```python
from build123d import *

# Parameters (mm, degrees)
MODEL_R                         = 1
MODEL_W                         = 12.3
MODEL_H                         = 22.500175579
BRIDA_BASE1_DEPTH               = 1
PLIEGUE_START                   = -94.948568727
PLIEGUE_CROQUIZADO1_DEPTH       = 36.500175579
PLIEGUE_CROQUIZADO1_2_DEPTH     = 2
PLIEGUE_START_2                 = -60.448393148
PLIEGUE_CROQUIZADO1_3_DEPTH     = 2
PLIEGUE_CROQUIZADO1_4_DEPTH     = 36.500175579
PLIEGUE_START_3                 = -92.948568727
PLIEGUE_CROQUIZADO1_5_DEPTH     = 32.500175579
PLIEGUE_START_4                 = 176.99991226
PLIEGUE_CROQUIZADO1_6_OUTLINE_R = 1
PLIEGUE_CROQUIZADO1_6_DEPTH     = 1


with BuildPart() as part:
    # Brida base1: sheet metal written as solids
    # Model → Brida base1 (new body)
    with BuildSketch(Plane.XY):
        with BuildLine():
            Line((178.265288891, -94.948568727), (178.265288891, -92.948568727))
            Line((178.265288891, -92.948568727), (177.265288891, -92.948568727))
            Line((177.265288891, -92.948568727), (177.265288891, -94.948568727))
            Line((177.265288891, -94.948568727), (169.565288891, -94.948568727))
            ThreePointArc((169.565288891, -94.948568727), (168.151075328, -94.362782289), (167.565288891, -92.948568727))
            Line((167.565288891, -92.948568727), (167.565288891, -60.448393148))
            ThreePointArc((167.565288891, -60.448393148), (168.151075328, -59.034179585), (169.565288891, -58.448393148))
            Line((169.565288891, -58.448393148), (177.265288891, -58.448393148))
            Line((177.265288891, -58.448393148), (177.265288891, -60.448393148))
            Line((177.265288891, -60.448393148), (178.265288891, -60.448393148))
            Line((178.265288891, -60.448393148), (178.265288891, -58.448393148))
            Line((178.265288891, -58.448393148), (195.565288891, -58.448393148))
            ThreePointArc((195.565288891, -58.448393148), (196.979502453, -59.034179585), (197.565288891, -60.448393148))
            Line((197.565288891, -60.448393148), (197.565288891, -92.948568727))
            ThreePointArc((197.565288891, -92.948568727), (196.979502453, -94.362782289), (195.565288891, -94.948568727))
            Line((195.565288891, -94.948568727), (178.265288891, -94.948568727))
        make_face()
        with Locations((171.565288891, -90.348568727)):
            Circle(MODEL_R, mode=Mode.SUBTRACT)
        with Locations((171.565288891, -63.048393148)):
            Circle(MODEL_R, mode=Mode.SUBTRACT)
        with Locations((188.165288891, -63.048393148)):
            Circle(MODEL_R, mode=Mode.SUBTRACT)
        with Locations((188.165288891, -90.348568727)):
            Circle(MODEL_R, mode=Mode.SUBTRACT)
        with Locations((188.415288891, -76.698480938)):
            Rectangle(MODEL_W, MODEL_H, mode=Mode.SUBTRACT)
    extrude(amount=-BRIDA_BASE1_DEPTH)

    # Pliegue croquizado1: read off the stored shape, not the designer's step
    # Pliegue croquizado1 outline → Pliegue croquizado1 (cut)
    with BuildSketch(Plane(origin=(0, 0, 0), x_dir=(1, 0, 0), z_dir=(0, 1, 0)).offset(PLIEGUE_START)):
        with BuildLine():
            Line((167.565288891, 0), (177.163871169, 0))
            ThreePointArc((177.163871169, 0), (177.804686096, 0.728828115), (178.73651226, 1))
            Line((178.73651226, 1), (167.565288891, 1))
            Line((167.565288891, 1), (167.565288891, 0))
        make_face()
    extrude(amount=PLIEGUE_CROQUIZADO1_DEPTH, mode=Mode.SUBTRACT)

    # Pliegue croquizado1 2 outline → Pliegue croquizado1 2 (cut)
    with BuildSketch(Plane(origin=(0, 0, 0), x_dir=(1, 0, 0), z_dir=(0, 1, 0)).offset(PLIEGUE_START)):
        with BuildLine():
            ThreePointArc((177.265288891, 0.186049099), (177.211739726, 0.094572835), (177.163871169, 0))
            Line((177.163871169, 0), (177.265288891, 0))
            Line((177.265288891, 0), (177.265288891, 0.186049099))
        make_face()
        Polygon((178.265288891, 0), (178.441395947, 0), (178.265288891, 0.439557056), align=None)
    extrude(amount=PLIEGUE_CROQUIZADO1_2_DEPTH, mode=Mode.SUBTRACT)

    # Pliegue croquizado1 3 outline → Pliegue croquizado1 3 (cut)
    with BuildSketch(Plane(origin=(0, 0, 0), x_dir=(1, 0, 0), z_dir=(0, 1, 0)).offset(PLIEGUE_START_2)):
        with BuildLine():
            ThreePointArc((177.265288891, 0.186049099), (177.211739726, 0.094572835), (177.163871169, 0))
            Line((177.163871169, 0), (177.265288891, 0))
            Line((177.265288891, 0), (177.265288891, 0.186049099))
        make_face()
        Polygon((178.265288891, 0), (178.441395947, 0), (178.265288891, 0.439557056), align=None)
    extrude(amount=PLIEGUE_CROQUIZADO1_3_DEPTH, mode=Mode.SUBTRACT)

    # Pliegue croquizado1 4 outline → Pliegue croquizado1 4 (add)
    with BuildSketch(Plane(origin=(0, 0, 0), x_dir=(1, 0, 0), z_dir=(0, 1, 0)).offset(PLIEGUE_START)):
        with BuildLine():
            Line((176.99991226, -9.965376631), (177.99991226, -9.965376631))
            Line((177.99991226, -9.965376631), (177.99991226, -0.7366))
            ThreePointArc((177.99991226, -0.7366), (178.01324203, -0.597101848), (178.0527489, -0.46265251))
            Line((178.0527489, -0.46265251), (177.124479337, -0.090744432))
            ThreePointArc((177.124479337, -0.090744432), (177.031338378, -0.407720702), (176.99991226, -0.7366))
            Line((176.99991226, -0.7366), (176.99991226, -9.965376631))
        make_face()
        with BuildLine():
            Line((178.441395947, 0), (178.462564769, -0.05283664))
            ThreePointArc((178.462564769, -0.05283664), (178.597014107, -0.01332977), (178.73651226, 0))
            Line((178.73651226, 0), (178.441395947, 0))
        make_face()
        with BuildLine():
            Line((178.090656691, 0.875432923), (178.265288891, 0.439557056))
            Line((178.265288891, 0.439557056), (178.265288891, 0.934844913))
            ThreePointArc((178.265288891, 0.934844913), (178.17718339, 0.907459237), (178.090656691, 0.875432923))
        make_face()
    extrude(amount=PLIEGUE_CROQUIZADO1_4_DEPTH)

    # Pliegue croquizado1 5 outline → Pliegue croquizado1 5 (add)
    with BuildSketch(Plane(origin=(0, 0, 0), x_dir=(1, 0, 0), z_dir=(0, 1, 0)).offset(PLIEGUE_START_3)):
        with BuildLine():
            Line((177.124479337, -0.090744432), (178.0527489, -0.46265251))
            ThreePointArc((178.0527489, -0.46265251), (178.215657405, -0.215745145), (178.462564769, -0.05283664))
            Line((178.462564769, -0.05283664), (178.441395947, 0))
            Line((178.441395947, 0), (177.163871169, 0))
            ThreePointArc((177.163871169, 0), (177.143528964, -0.045091664), (177.124479337, -0.090744432))
        make_face()
    extrude(amount=PLIEGUE_CROQUIZADO1_5_DEPTH)

    # Pliegue croquizado1 6 outline → Pliegue croquizado1 6 (cut)
    with BuildSketch(Plane.YZ.offset(PLIEGUE_START_4)):
        with BuildLine():
            Line((-58.448393148, 9.965376631), (-60.448393148, 9.965376631))
            ThreePointArc((-60.448393148, 9.965376631), (-59.034179585, 9.379590194), (-58.448393148, 7.965376631))
            Line((-58.448393148, 7.965376631), (-58.448393148, 9.965376631))
        make_face()
        with BuildLine():
            ThreePointArc((-94.948568727, 7.965376631), (-94.362782289, 9.379590194), (-92.948568727, 9.965376631))
            Line((-92.948568727, 9.965376631), (-94.948568727, 9.965376631))
            Line((-94.948568727, 9.965376631), (-94.948568727, 7.965376631))
        make_face()
        with Locations((-90.348568727, 5.965376631)):
            Circle(PLIEGUE_CROQUIZADO1_6_OUTLINE_R)
        with Locations((-63.048393148, 5.965376631)):
            Circle(PLIEGUE_CROQUIZADO1_6_OUTLINE_R)
    extrude(amount=PLIEGUE_CROQUIZADO1_6_DEPTH, mode=Mode.SUBTRACT)


solid = part.part
```
Model file for the job. Use its own axes, mm. A direction names the side the tool comes from. Round coordinates to 2 decimals unless told otherwise and drop trailing zeros. Loops run counter-clockwise (first coordinate to the right, second up) from the corner with the lowest first, then second, coordinate; pieces in that order, holes last. Notation, with made-up numbers: M 2.25,63.25 L 38.25,63.25 A8 ccw 38.25,68.25 Z; hole C -31,-33.75 d11. An arc over 180 degrees is marked long. Put each result on its own line as item: value. Start each with the question number.
Item 1: Cut at D-D (z = 6.5). List the corners of the cut face in (x, y).
Item 2: Drill centre lines: line 1 along X through (y, z) = (-69, 2.25); line 2 along Z through (x, y) = (186.5, -61). Where is each one in solid material? Low to high.
Item 3: Cut at B-B (x = 183.5). List the corners of the cut face in (y, z).
Item 4: Mould opens along X. For faces 1 (the face through (177.6, -59.46, 0.28)), 2 (the face through (177.49, -94.38, 9.36)), 3 (the face through (188.3, -65.448, -0.5)) say: released by +X, released by -X, zero draft, split by the parting line, or undercut.
Item 5: Cut at A-A (y = -85.5). List the corners of the cut face in (x, z).
Item 6: Drop flat-ended pins along their axis: P1, Ø4.5, axis at y = -84.5, z = 7.5, coming from the +X side; P2, Ø1.5, axis at x = 183.5, y = -63, coming from the +Z side; P3, Ø1.1, axis at y = -77, z = -0.5, coming from the -X side. Give the stop position or say it passes through.
Item 7: Cut at C-C (y = -65). List the corners of the cut face in (x, z), then the cut area to 3 significant figures.
Item 8: 3-axis set-ups, long thin cutter, end or side, ignore diameter. For faces 4 (the face through (194.565, -76.9, -0.5)), 5 (the face through (177.6, -93.96, 0.28)), 6 (the face through (178, -92.949, 0)): which of +Z, -Z, +X, -X, +Y, -Y reach the whole face in a straight line?
Answer block:
1. outline: M 177,-94.95 L 178,-94.95 L 178,-91.19 L 177,-91.19 Z; M 177,-89.5 L 178,-89.5 L 178,-63.89 L 177,-63.89 Z; M 177,-62.2 L 178,-62.2 L 178,-58.45 L 177,-58.45 Z
2. line 1: 177 to 178
2. line 2: -1 to 0
3. outline: M -94.95,-1 L -87.95,-1 L -87.95,0 L -94.95,0 Z; M -65.45,-1 L -58.45,-1 L -58.45,0 L -65.45,0 Z
4. face 1: released by +X
4. face 2: zero draft
4. face 3: undercut
5. outline: M 177,0.74 A1.74 ccw 178.74,-1 L 182.27,-1 L 182.27,0 L 178.74,0 A0.74 cw 178,0.74 L 178,9.97 L 177,9.97 Z; M 194.57,-1 L 197.57,-1 L 197.57,0 L 194.57,0 Z
6. P1: x = 178
6. P2: z = 0
6. P3: x = 177.14
7. outline: M 177,0.74 A1.74 ccw 178.74,-1 L 197.57,-1 L 197.57,0 L 178.74,0 A0.74 cw 178,0.74 L 178,9.97 L 177,9.97 Z
7. area: 30.0 mm2
8. face 4: +Z, -Z
8. face 5: -Z, +X, -Y
8. face 6: -Y
